Here's how the part is built. I have some questions about the finished solid (model axes, mm). Round coordinates to 2 decimals unless told otherwise and drop trailing zeros. Loops run counter-clockwise (first coordinate to the right, second up) from the corner with the lowest first, then second, coordinate; pieces in that order, holes last. Notation, with made-up numbers: M -12.5,63.5 L 13.5,63.5 A24 ccw 13.5,88.5 Z; hole C -28,-15 d7. An arc over 180 degrees is marked long. Answer as a JSON object with one key per item and string values.
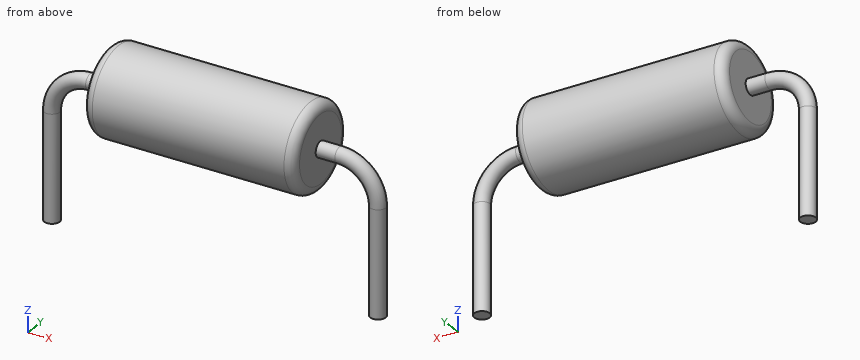
from build123d import *

# Parameters (mm, degrees)
SKETCH_3_R      = 2.25
EXTRUDE_1_DEPTH = 11
SKETCH_4_R      = 0.4
FILLET_1_R      = 0.5


with BuildPart() as part:
    # Эскиз3 → Вытянуть1 (new body)
    with BuildSketch(Plane(origin=(3, 0, 0), x_dir=(0, 0, -1), z_dir=(1, 0, 0))):
        with Locations((-2.25, 0)):
            Circle(SKETCH_3_R)
    extrude(amount=EXTRUDE_1_DEPTH)

    # По траектории1: sweep along a path in Эскиз5
    with BuildLine(Plane(origin=(0, 0, 0), x_dir=(1, 0, 0), z_dir=(0, 1, 0))) as sweep_1_path:
        Line((0, 5.25), (0, -0.25))
        ThreePointArc((0, -0.25), (0.585786438, -1.664213562), (2, -2.25))
        Line((2, -2.25), (2.965757317, -2.25))
        Line((2.965757317, -2.25), (14, -2.25))
        Line((14, -2.25), (15, -2.25))
        ThreePointArc((15, -2.25), (16.414213562, -1.664213562), (17, -0.25))
        Line((17, -0.25), (17, 0))
        Line((17, 0), (17, 5.250003271))
    # Эскиз4 → По траектории1 (sweep)
    with BuildSketch(Plane.XY.offset(-5.25)):
        Circle(SKETCH_4_R)
    sweep(path=sweep_1_path.line)

    # Скругление1
    fillet_1_edges = [part.edges().sort_by_distance(p)[0] for p in [
        (3, 0, 4.5),
        (14, 0, 4.5),
    ]]
    fillet(fillet_1_edges, radius=FILLET_1_R)


solid = part.part
Item 1: I want a section at C-C, the plane x = 7.25. Please give me the cut outline in (y, z).
Resolved:
{"outline": "C 0,2.25 d4.5"}
Item 2: I want a section at B-B, the plane z = -1.25. Please give me the cut outline in (x, y), then the cut area to 3 significant figures.
Resolved:
{"outline": "C 0,0 d0.8; C 17,0 d0.8", "area": "1.01 mm²"}
Item 3: I'm going to push flat-ended pins straight in: pin 1 Ø3 at (x, z) = (15, -4) entering from +Y; pin 2 Ø2 at (x, z) = (9, 1) entering from +Y; pin 3 Ø2 at (x, z) = (14, 3.5) entering from -Y. Where does each tip first touch, or does it pass through?
Resolved:
{"pin 1": "through", "pin 2": "y = 2.24", "pin 3": "y = -2.22"}
Item 4: Please list where these lines run through material, in increasing order: probe 1 along X at (y, z) = (0.15, 0.75); probe 2 along X at (y, z) = (-1.2, 3.25); probe 3 along X at (y, z) = (0.1, -3.5). Write a range as from..to.
Resolved:
{"probe 1": "-0.32..0.45, 3..14, 16.55..17.32", "probe 2": "3..14", "probe 3": "-0.39..0.39, 16.61..17.39"}
Item 5: I want a section at A-A, the plane y = 0. Please give me the cut outline in (x, z).
Resolved:
{"outline": "M -0.4,-5.25 L 0.4,-5.25 L 0.4,0.25 A1.6 cw 2,1.85 L 3,1.85 L 3,0.5 A0.5 ccw 3.5,0 L 13.5,0 A0.5 ccw 14,0.5 L 14,1.85 L 15,1.85 A1.6 cw 16.6,0.25 L 16.6,-5.25 L 17.4,-5.25 L 17.4,0.25 A2.4 ccw 15,2.65 L 14,2.65 L 14,4 A0.5 ccw 13.5,4.5 L 3.5,4.5 A0.5 ccw 3,4 L 3,2.65 L 2,2.65 A2.4 ccw -0.4,0.25 Z"}
